Work out the finished part from the listing and answer in its coordinate system (mm). Face numbers are marked on the shaded views. A direction names the side the tool comes from. Give positions to 0.01 mm unless a question says otherwise; leave off trailing zeros. Loops run counter-clockwise (first coordinate to the right, second up) from the corner with the lowest first, then second, coordinate; pieces in that order, holes last. Notation, with made-up numbers: M 87.5,-7 L 144.5,-7 A21 ccw 144.5,1 Z; hole C 40.5,10.25 d10. An arc over 180 degrees is marked long. Use a Markdown table: item, result.
```python
from build123d import *

# Parameters (mm, degrees)
F0_R     = 3
F1_DEPTH = 14


with BuildPart() as f1:
    # F0 (on Front) → F1 (new body)
    with BuildSketch(Plane.XZ):
        with BuildLine():
            Line((-20, 8), (-32, 8))
            ThreePointArc((-32, 8), (-40, 0), (-32, -8))
            Line((-32, -8), (0, -8))
            ThreePointArc((0, -8), (8, 0), (0, 8))
            Line((0, 8), (0, 16))
            Line((0, 16), (-20, 16))
            Line((-20, 16), (-20, 8))
        make_face()
        with Locations((-32, 0)):
            Circle(F0_R, mode=Mode.SUBTRACT)
        Circle(F0_R, mode=Mode.SUBTRACT)
    extrude(amount=F1_DEPTH)


solid = f1.part
```
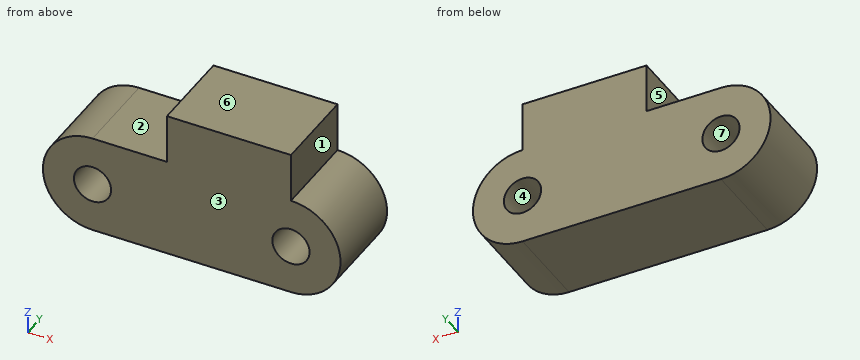
(1) Given P1, Ø8, axis at x = 0, z = 0, coming from the -Y side; P2, Ø4, axis at y = -4, z = 12, coming from the +X side; P3, Ø3.5, axis at x = -23.5, y = -7.5, coming from the +Z side; P4, Ø2.5, axis at y = -4.5, z = 10.5, coming from the -X side, each flat-ended and moving along its own axis, determine where each tip first touches the part or whether it passes through.
Entries:
| item | result |
|---|---|
| P1 | stops at y = -14 |
| P2 | stops at x = 0 |
| P3 | stops at z = 8 |
| P4 | stops at x = -20 |
(2) A cutting plane is placed at D-D (z = -2.5). Write down the section's boundary in (x, y).
Entries:
| item | result |
|---|---|
| outline | M -39.6,-14 L -33.66,-14 L -33.66,0 L -39.6,0 Z; M -30.34,-14 L -1.66,-14 L -1.66,0 L -30.34,0 Z; M 1.66,-14 L 7.6,-14 L 7.6,0 L 1.66,0 Z |
(3) The mould has two halves that part along X. Classify the marked faces 4, 5, 6 and 7: released by +X, released by -X, zero draft, split by the parting line, or undercut.
Entries:
| item | result |
|---|---|
| face 4 | undercut |
| face 5 | released by -X |
| face 6 | zero draft |
| face 7 | undercut |
(4) A cutting plane is placed at A-A (z = 0). Write down the section's boundary in (x, y).
Entries:
| item | result |
|---|---|
| outline | M -40,-14 L -35,-14 L -35,0 L -40,0 Z; M -29,-14 L -3,-14 L -3,0 L -29,0 Z; M 3,-14 L 8,-14 L 8,0 L 3,0 Z |
(5) A cutting plane is placed at C-C (x = -27). Write down the section's boundary in (y, z), and give its area (3 significant figures).
Entries:
| item | result |
|---|---|
| outline | M -14,-8 L 0,-8 L 0,8 L -14,8 Z |
| area | 224 mm² |
(6) Consider probe 1 along Z at (x, y) = (-32, -5.25); probe 2 along X at (y, z) = (-5, 0.25); probe 3 along X at (y, z) = (-10.5, -1.5). Determine where each line is inside the solid, lowest interval first. Write a range as [from, to].
Entries:
| item | result |
|---|---|
| probe 1 | z = [-8, -3], [3, 8] |
| probe 2 | x = [-40, -34.99], [-29.01, -2.99], [2.99, 8] |
| probe 3 | x = [-39.86, -34.6], [-29.4, -2.6], [2.6, 7.86] |
(7) A cutting plane is placed at B-B (y = -3.25). Write down the section's boundary in (x, z).
Entries:
| item | result |
|---|---|
| outline | M -32,-8 L 0,-8 A8 ccw 0,8 L 0,16 L -20,16 L -20,8 L -32,8 A8 ccw Z; hole C -32,0 d6; hole C 0,0 d6 |
(8) Which of the six approach directions +Z, -Z, +X, -X, +Y, -Y give full straight-line access (tool end or side, diameter ignored) to the marked faces 1, 2 and 3?
Entries:
| item | result |
|---|---|
| face 1 | +Z, +X, +Y, -Y |
| face 2 | +Z, -X, +Y, -Y |
| face 3 | +Z, -Z, +X, -X, -Y |
